```python
from build123d import *

# Parameters (mm, degrees)
F1_R     = 19.907119
F2_DEPTH = 12.7
F3_R     = 14.872727
F4_DEPTH = 19.05
F0_R     = 11.75258
F5_DEPTH = 8.89


with BuildPart() as f2:
    # F1 (on Top) → F2 (new body)
    with BuildSketch(Plane.XY):
        Circle(F1_R)
    extrude(amount=-F2_DEPTH)

    # F3 (on Top) → F4 (join)
    with BuildSketch(Plane.XY):
        Circle(F3_R)
    extrude(amount=-F4_DEPTH)

    # F0 (on Top) → F5 (cut)
    with BuildSketch(Plane.XY):
        Circle(F0_R)
    extrude(amount=-F5_DEPTH, mode=Mode.SUBTRACT)


solid = f2.part
```
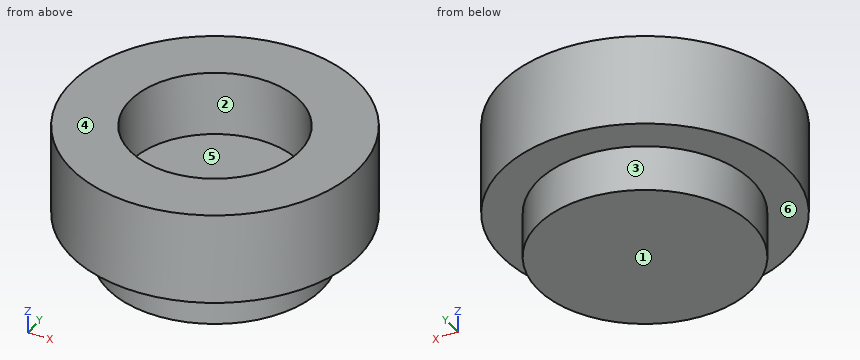
The listing builds one solid part. Answer for the finished solid, in the listing's coordinates (mm). Face numbers are marked on the shaded views. A direction names the side the tool comes from. Give positions to 0.01 mm unless a question says otherwise; leave off trailing zeros. Loops run counter-clockwise (first coordinate to the right, second up) from the corner with the lowest first, then second, coordinate; pieces in that order, holes last. Notation, with made-up numbers: M 89.25,15.5 L 109.25,15.5 A23 ccw 109.25,33.5 Z; hole C 24,40 d1. An arc over 180 degrees is marked long. One line per item, written item: value.
Q1. A cutting plane is placed at A-A on x = 0. Determine the outline of the cut face in (y, z).
Working result:
outline: M -19.91,-12.7 L -14.87,-12.7 L -14.87,-19.05 L 14.87,-19.05 L 14.87,-12.7 L 19.91,-12.7 L 19.91,0 L 11.75,0 L 11.75,-8.89 L -11.75,-8.89 L -11.75,0 L -19.91,0 Z
Q2. A cutting plane is placed at C-C on z = -9.75. Determine the outline of the cut face in (x, y), then the cut area to 3 significant figures.
Working result:
outline: C 0,0 d39.81
area: 1,240 mm^2
Q3. A cutting plane is placed at D-D on z = -3.5. Determine the outline of the cut face in (x, y).
Working result:
outline: C 0,0 d39.81; hole C 0,0 d23.51
Q4. Determine the mould class of the marked faces 1, 2 and 3 for opening direction X: +X half, -X half, draft (parallel to the pull), parting line (faces both ways), or undercut.
Working result:
face 1: draft
face 2: undercut
face 3: parting line
Q5. Flat-ended cylindrical pins translate along their axes: P1, Ø5, axis at x = 0, y = -4.5, coming from the +Z side; P2, Ø2, axis at y = -9, z = -12, coming from the -X side; P3, Ø1, axis at x = -13, z = -14, coming from the -Y side. Find the tip coordinate at first contact, or state that the pin passes through.
Working result:
P1: stops at z = -8.89
P2: stops at x = -18.23
P3: stops at y = -8.06
Q6. Find the intervals of material crossed by line 1 (Y direction, x = 0, z = -7); line 2 (Z direction, x = 4.5, y = -16); line 3 (Z direction, x = 5.5, y = -9), in increasing order. Write a range as from..to.
Working result:
line 1: y = -19.91..-11.75, 11.75..19.91
line 2: z = -12.7..0
line 3: z = -19.05..-8.89
Q7. For the marked faces 4, 5 and 6, determine the directions among +Z, -Z, +X, -X, +Y, -Y from which every point of the face is accessible in a straight line to the end or side of a thin tool.
Working result:
face 4: +Z, +X, -X, +Y, -Y
face 5: +Z
face 6: -Z
